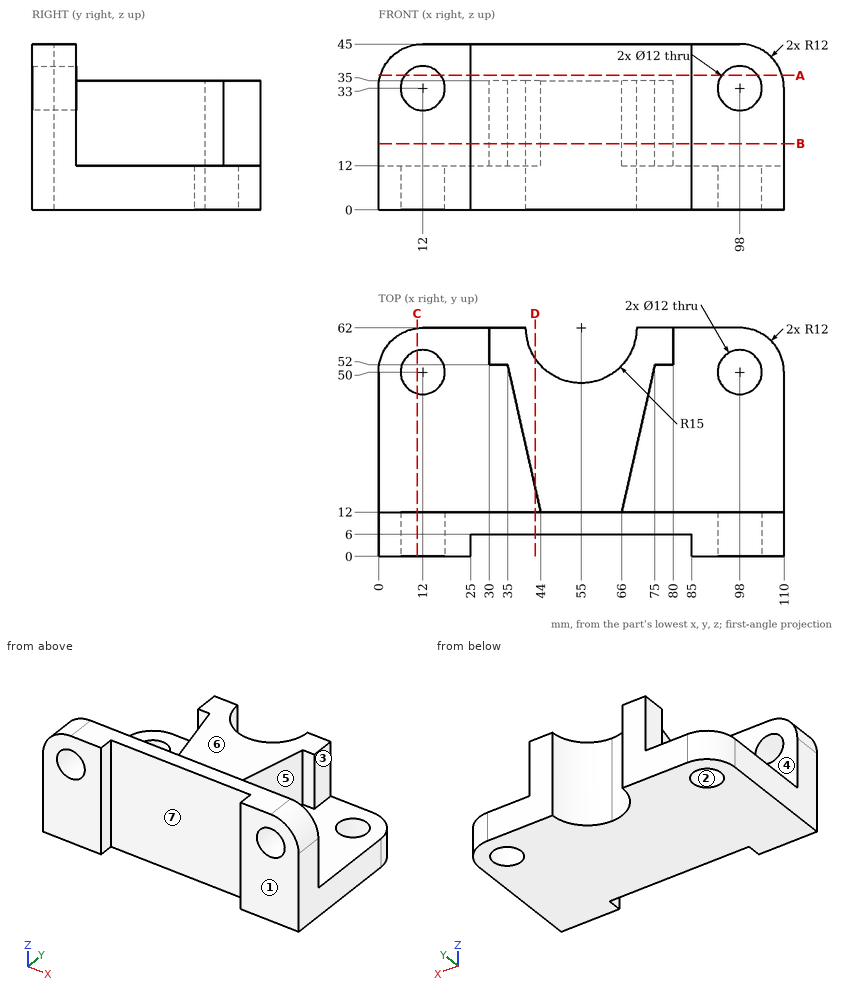
Geometry check sheet. Reference: drawing and pictorial views, mm from the part's lowest x, y, z. A direction names the side the tool comes from. Coordinates: 2 decimals unless noted, no trailing zeros. Loops run counter-clockwise (first coordinate to the right, second up) from the corner with the lowest first, then second, coordinate; pieces in that order, holes last. Notation, with made-up numbers: (63, 33.25) -> (106, 33.25) arc R21 ccw to (106, 56.25) -> close; hole circle Ø5 at (22.25, 72.5). An arc over 180 degrees is marked (long way). Put each result on its own line as item: value.
1) Tool access check on the marked faces 4, 5, 6 and 7. Record the directions out of +Z, -Z, +X, -X, +Y, -Y that give a thin tool (end or side, any length) a straight path to the whole face; none if there is none.
Result set:
face 4: +Z
face 5: +Z, +X
face 6: +Z, +X, -X, +Y
face 7: +Z, -Z, -Y
2) Cross-section at C-C on x = 10.5. Record the boundary of the cut face in (y, z), plus the area to 3 significant figures.
Result set:
outline: (0, 0) -> (44.19, 0) -> (44.19, 12) -> (12, 12) -> (12, 27.19) -> (0, 27.19) -> close; (0, 38.81) -> (12, 38.81) -> (12, 44.91) -> (0, 44.91) -> close; (55.81, 0) -> (61.91, 0) -> (61.91, 12) -> (55.81, 12) -> close
area: 859 mm^2
3) Thickness scan on line 1 (X direction, y = 7, z = 33); line 2 (Y direction, x = 32, z = 23); line 3 (Z direction, x = 12, y = 4.25). Record the ranges inside material, lowest first.
Result set:
line 1: x = 0 to 6, 18 to 92, 104 to 110
line 2: y = 6 to 12, 52 to 62
line 3: z = 0 to 27, 39 to 45
4) Release check for a two-part mould opening along Y. For the marked faces 1, 2 and 3 record: released by +Y, released by -Y, zero draft, split by the parting line, or undercut.
Result set:
face 1: released by -Y
face 2: undercut
face 3: zero draft
5) Gauge pin test, flat ends, axial feed: pin 1 Ø22 at (x, y) = (78, 49.5) entering from +Z; pin 2 Ø22.5 at (x, z) = (59, 20) entering from -Y; pin 3 Ø7 at (x, y) = (98, 50) entering from +Z; pin 4 Ø8 at (y, z) = (55.5, 24.5) entering from +X. Record the tip position at first contact, or that the pin passes through.
Result set:
pin 1: stops at z = 35
pin 2: stops at y = 6
pin 3: passes through
pin 4: stops at x = 80
6) Cross-section at A-A on z = 36.5. Record the boundary of the cut face in (x, y).
Result set:
outline: (0.52, 0) -> (7.13, 0) -> (7.13, 12) -> (0.52, 12) -> close; (16.87, 0) -> (25, 0) -> (25, 6) -> (85, 6) -> (85, 0) -> (93.13, 0) -> (93.13, 12) -> (16.87, 12) -> close; (102.87, 0) -> (109.48, 0) -> (109.48, 12) -> (102.87, 12) -> close
7) Cross-section at D-D on x = 42.5. Record the boundary of the cut face in (y, z), plus the area to 3 significant figures.
Result set:
outline: (6, 0) -> (53.71, 0) -> (53.71, 35) -> (18.67, 35) -> (18.67, 12) -> (12, 12) -> (12, 45) -> (6, 45) -> close
area: 1,580 mm^2
8) Cross-section at B-B on z = 18. Record the boundary of the cut face in (x, y), plus the area to 3 significant figures.
Result set:
outline: (0, 0) -> (25, 0) -> (25, 6) -> (85, 6) -> (85, 0) -> (110, 0) -> (110, 12) -> (66, 12) -> (75, 52) -> (80, 52) -> (80, 62) -> (70, 62) arc R15 cw to (40, 62) -> (30, 62) -> (30, 52) -> (35, 52) -> (44, 12) -> (0, 12) -> close
area: 2,350 mm^2
